from build123d import *

# Parameters (mm, degrees)
SKETCH1_W           = 33.4
SKETCH1_H           = 20.4
BOSS_EXTRUDE1_DEPTH = 3
SKETCH4_R           = 1.27
CUT_EXTRUDE1_DEPTH  = 40.252006318
FILLET5_R           = 3


with BuildPart() as part:
    # Sketch1 → Boss-Extrude1 (new body)
    with BuildSketch(Plane(origin=(0, 0, 0), x_dir=(1, 0, 0), z_dir=(0, 1, 0))):
        with Locations((16.7, 10.2)):
            Rectangle(SKETCH1_W, SKETCH1_H)
    extrude(amount=BOSS_EXTRUDE1_DEPTH)

    # Sketch4 → Cut-Extrude1 (cut, through all)
    with BuildSketch(Plane(origin=(0, 3, 0), x_dir=(1, 0, 0), z_dir=(0, 1, 0))):
        with Locations(Location((2.54, 17.86, 0), (0, 0, 270))):
            Circle(SKETCH4_R)
        with Locations(Location((2.54, 2.54, 0), (0, 0, 270))):
            Circle(SKETCH4_R)
        with Locations(Location((30.86, 17.86, 0), (0, 0, 270))):
            Circle(SKETCH4_R)
        with Locations(Location((30.86, 2.54, 0), (0, 0, 270))):
            Circle(SKETCH4_R)
    extrude(amount=-CUT_EXTRUDE1_DEPTH, mode=Mode.SUBTRACT)

    # Fillet5
    fillet5_edges = [part.edges().sort_by_distance(p)[0] for p in [
        (0, 1.5, 0),
        (0, 1.5, -20.4),
        (33.4, 1.5, -20.4),
        (33.4, 1.5, 0),
    ]]
    fillet(fillet5_edges, radius=FILLET5_R)


solid = part.part
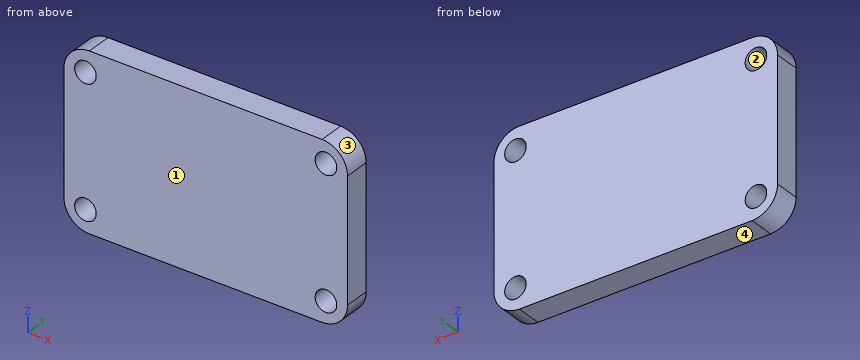
Geometry check sheet. Reference: the model listing, model coordinates, mm. Face numbers are marked on the shaded views. Give positions to 0.01 mm unless a question says otherwise; leave off trailing zeros. Loops run counter-clockwise (first coordinate to the right, second up) from the corner with the lowest first, then second, coordinate; pieces in that order, holes last. Notation, with made-up numbers: M -29.75,61.5 L -17.75,61.5 A17 cw -17.75,84.5 Z; hole C 15,73 d1. An arc over 180 degrees is marked long. Answer as a JSON object with one key per item and string values. Group by question number.
Item 1: Sectioned sample at C-C on x = 2.54. Record the boundary of the cut face in (y, z).
Item 2: Sectioned sample at A-A on y = 2. Record the boundary of the cut face in (x, z).
Item 3: Sectioned sample at B-B on z = -2.54. Record the boundary of the cut face in (x, y).
Item 4: Mould release check, pull along Z, two halves, no side actions. Record for the marked faces 1, 2, 3 and 4: pulls with the +Z half, pulls with the -Z half, needs draft (parallel to the pull), parting line crosses it, or undercut.
Item 5: Material ranges on L1, parallel to X at y = 2, z = -17.86; L2, parallel to Z at x = 31, y = 0.55; L3, parallel to X at y = 2.6, z = -18.5, recorded low to high.
Findings below:
{
 "1": {"outline": "M 0,-20.36 L 3,-20.36 L 3,-19.13 L 0,-19.13 Z; M 0,-16.59 L 3,-16.59 L 3,-3.81 L 0,-3.81 Z; M 0,-1.27 L 3,-1.27 L 3,-0.04 L 0,-0.04 Z"},
 "2": {"outline": "M 0,-17.4 A3 ccw 3,-20.4 L 30.4,-20.4 A3 ccw 33.4,-17.4 L 33.4,-3 A3 ccw 30.4,0 L 3,0 A3 ccw 0,-3 Z; hole C 2.54,-17.86 d2.54; hole C 2.54,-2.54 d2.54; hole C 30.86,-17.86 d2.54; hole C 30.86,-2.54 d2.54"},
 "3": {"outline": "M 0.04,0 L 1.27,0 L 1.27,3 L 0.04,3 Z; M 3.81,0 L 29.59,0 L 29.59,3 L 3.81,3 Z; M 32.13,0 L 33.36,0 L 33.36,3 L 32.13,3 Z"},
 "4": {"face 1": "needs draft", "face 2": "undercut", "face 3": "pulls with the +Z half", "face 4": "pulls with the -Z half"},
 "5": {"L1": "0.04 to 1.27, 3.81 to 29.59, 32.13 to 33.36", "L2": "-20.34 to -19.12, -16.6 to -3.8, -1.28 to -0.06", "L3": "0.21 to 1.44, 3.64 to 29.76, 31.96 to 33.19"}
}
